from build123d import *

# Parameters (mm, degrees)
IZIM1_W                     = 200
IZIM1_H                     = 150
Y_KSEKLIK_EKSTR_ZYON1_DEPTH = 30
Y_KSEKLIK_EKSTR_ZYON1_TAPER = 21
IZIM2_W                     = 159.102427113
IZIM2_H                     = 106.722832774
KES_EKSTR_ZYON1_DEPTH       = 5


with BuildPart() as part:
    # Çizim1 → Yükseklik-Ekstrüzyon1 (new body)
    with BuildSketch(Plane.XY):
        with Locations((100, 75)):
            Rectangle(IZIM1_W, IZIM1_H)
    extrude(amount=Y_KSEKLIK_EKSTR_ZYON1_DEPTH, taper=Y_KSEKLIK_EKSTR_ZYON1_TAPER)

    # Çizim2 → Kes-Ekstrüzyon1 (cut)
    with BuildSketch(Plane.XY.offset(30)):
        with Locations((101.653948212, 73.301492912)):
            Rectangle(IZIM2_W, IZIM2_H)
    extrude(amount=-KES_EKSTR_ZYON1_DEPTH, mode=Mode.SUBTRACT)


solid = part.part
Work out the finished part from the listing and answer in its coordinate system (mm). A direction names the side the tool comes from. Give positions to 0.01 mm unless a question says otherwise; leave off trailing zeros. Loops run counter-clockwise (first coordinate to the right, second up) from the corner with the lowest first, then second, coordinate; pieces in that order, holes last. Notation, with made-up numbers: (64, 46) -> (99, 46) arc R16 cw to (99, 70) -> close; hole circle Ø6 at (-17.5, 18). An arc over 180 degrees is marked (long way). Use a Markdown table: item, result. Add a question column.
1) Consider line 1 along Z through (x, y) = (47, 100); line 2 along X through (y, z) = (62.5, 28); line 3 along X through (y, z) = (57, 25.5). Determine where each line is inside the solid, lowest interval first.
2) Which of the six approach directions +Z, -Z, +X, -X, +Y, -Y give full straight-line access (tool end or side, diameter ignored) to faces 1 (the flat face through (101, 126.663, 28)), 2 (the flat face through (99, 76, 0))?
3) The part is cut by section A-A, the plane x = 142. Determine the outline of the cut face in (y, z), plus the area to 3 significant figures.
4) Each of these flat-tipped pins is pushed along its axis until it touches: P1, Ø1.5, axis at y = 38.5, z = 7.5, coming from the -X side; P2, Ø5.5, axis at y = 64, z = 28, coming from the -X side; P3, Ø8, axis at x = 74.5, z = 5, coming from the -Y side. Where does it stop, or does it pass through?
5) The part is cut by section C-C, the plane z = 11.5. Determine the outline of the cut face in (x, y).
6) For a pull along X with two mould halves and no side action, classify faces 3 (the flat face through (86, 127, 30)), 4 (the flat face through (194.323, 76.05, 14.79)), 5 (the flat face through (101, 19.94, 28)) as +X half, -X half, draft (parallel to the pull), parting line (faces both ways), or undercut.
7) The part is cut by section D-D, the plane y = 134. Determine the outline of the cut face in (x, z).
8) The part is cut by section B-B, the plane y = 90. Determine the outline of the cut face in (x, z).
Reported:
| question | item | result |
|---|---|---|
| 1 | line 1 | z = 0 to 25 |
| 1 | line 2 | x = 10.75 to 22.1, 181.21 to 189.25 |
| 1 | line 3 | x = 9.79 to 22.1, 181.21 to 190.21 |
| 2 | face 1 | +Z |
| 2 | face 2 | -Z, +X, -X, +Y, -Y |
| 3 | outline | (0, 0) -> (150, 0) -> (138.48, 30) -> (126.66, 30) -> (126.66, 25) -> (19.94, 25) -> (19.94, 30) -> (11.52, 30) -> close |
| 3 | area | 3,620 mm^2 |
| 4 | P1 | stops at x = 2.59 |
| 4 | P2 | stops at x = 9.69 |
| 4 | P3 | stops at y = 0.38 |
| 5 | outline | (4.41, 4.41) -> (195.59, 4.41) -> (195.59, 145.59) -> (4.41, 145.59) -> close |
| 6 | face 3 | draft |
| 6 | face 4 | +X half |
| 6 | face 5 | undercut |
| 7 | outline | (0, 0) -> (200, 0) -> (188.48, 30) -> (11.52, 30) -> close |
| 8 | outline | (0, 0) -> (200, 0) -> (188.48, 30) -> (181.21, 30) -> (181.21, 25) -> (22.1, 25) -> (22.1, 30) -> (11.52, 30) -> close |
